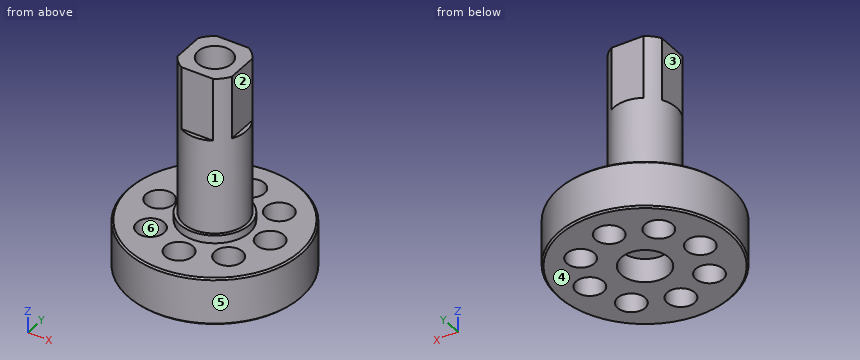
from build123d import *

# Parameters (mm, degrees)
F0_R      = 11
F1_DEPTH  = 6
F2_R      = 4
F3_DEPTH  = 21
F4_R      = 4.4
F5_DEPTH  = 1
F6_W      = 10
F6_H      = 10
F6_W_2    = 6.9
F6_H_2    = 6.9
F7_DEPTH  = 8
F8_R      = 1.75
F9_DEPTH  = 25
F11_SIZE  = 0.2
F12_R     = 2.15
F13_DEPTH = 10
F10_R     = 3
F14_DEPTH = 3


with BuildPart() as f1:
    # F0 (on Top) → F1 (new body)
    with BuildSketch(Plane.XY):
        Circle(F0_R)
    extrude(amount=F1_DEPTH)

    # F2 (on face) → F3 (join)
    with BuildSketch(Plane.XY.offset(6)):
        Circle(F2_R)
    extrude(amount=F3_DEPTH)

    # F4 (on face) → F5 (join)
    with BuildSketch(Plane.XY.offset(6)):
        Circle(F4_R)
    extrude(amount=F5_DEPTH)

    # F6 (on face) → F7 (cut)
    with BuildSketch(Plane.XY.offset(27)):
        Rectangle(F6_W, F6_H)
        Rectangle(F6_W_2, F6_H_2, mode=Mode.SUBTRACT)
    extrude(amount=-F7_DEPTH, mode=Mode.SUBTRACT)

    # F8 (on face) → F9 (cut)
    with BuildSketch(Plane(origin=(0, 0, 0), x_dir=(1, 0, 0), z_dir=(0, 0, -1))):
        with Locations((0, 7)):
            Circle(F8_R)
        with Locations((-4.949747, 4.949747)):
            Circle(F8_R)
        with Locations((-7, 0)):
            Circle(F8_R)
        with Locations((-4.949747, -4.949747)):
            Circle(F8_R)
        with Locations((0, -7)):
            Circle(F8_R)
        with Locations((4.949747, -4.949747)):
            Circle(F8_R)
        with Locations((7, 0)):
            Circle(F8_R)
        with Locations((4.949747, 4.949747)):
            Circle(F8_R)
    extrude(amount=-F9_DEPTH, mode=Mode.SUBTRACT)

    # F11
    f11_edges = [f1.edges().sort_by_distance(p)[0] for p in [
        (11, 0, 3),
        (-11, 0, 0),
        (-11, 0, 6),
    ]]
    chamfer(f11_edges, length=F11_SIZE)

    # F12 (on face) → F13 (cut)
    with BuildSketch(Plane.XY.offset(27)):
        Circle(F12_R)
    extrude(amount=-F13_DEPTH, mode=Mode.SUBTRACT)

    # F10 (on face) → F14 (cut)
    with BuildSketch(Plane(origin=(0, 0, 0), x_dir=(1, 0, 0), z_dir=(0, 0, -1))):
        Circle(F10_R)
    extrude(amount=-F14_DEPTH, mode=Mode.SUBTRACT)


solid = f1.part
For this review, take the finished solid that the model builds, in its own axes (mm). Face numbers are marked on the shaded views. A direction names the side the tool comes from. Round coordinates to 2 decimals unless told otherwise and drop trailing zeros. Write each loop counter-clockwise with the first axis right and the second up, starting at its lowest first coordinate (ties: lowest second). Pieces come first, ordered by that corner, then holes. Notation, with made-up numbers: (14, -39) -> (48, -39) arc R13 cw to (48, -20) -> close; hole circle Ø5 at (88, -39). An arc over 180 degrees is marked (long way). Put each result on its own line as item: value.
Q1. The part is to be moulded in two halves that separate along X. For the marked faces 4, 5 and 6, say which applies: released by +X, released by -X, zero draft, split by the parting line, or undercut.
Determined:
face 4: zero draft
face 5: split by the parting line
face 6: undercut
Q2. Clearance check with flat-ended pins moving along their axes: pin 1 Ø2 at (x, y) = (-0.5, 0.5) entering from +Z; pin 2 Ø3 at (x, z) = (0.5, 22.5) entering from -Y; pin 3 Ø12 at (x, z) = (5, 21.5) entering from +Y; pin 4 Ø3 at (x, y) = (-4.95, -4.95) entering from -Z. State where each tip first meets the part, or that it passes through.
Determined:
pin 1: stops at z = 17
pin 2: stops at y = -3.45
pin 3: stops at y = 4
pin 4: passes through
Q3. Machinability: for the marked faces 1, 2 and 3, which of the approach directions +Z, -Z, +X, -X, +Y, -Y give a long, thin tool a straight path to every point of the face, cutting with its end or side? Answer none if there is none.
Determined:
face 1: +Z
face 2: +Z, +X, +Y, -Y
face 3: +Z, -X, +Y, -Y
Q4. To check wall thickness, follow L1, parallel to Y at x = 0, z = 4.75; L2, parallel to Y at x = 7, z = 1.9; L3, parallel to Z at x = -2.75, y = -6.25. State the ranges of each line that lie inside material, in increasing order. Write a range as [from, to].
Determined:
L1: y = [-11, -8.75], [-5.25, 5.25], [8.75, 11]
L2: y = [-8.49, -1.75], [1.75, 8.49]
L3: z = [0, 6]
Q5. Consider section A-A on z = 24.25. State the section outline as (x, y) points.
Determined:
outline: (-3.45, -2.02) arc R4 ccw to (-2.02, -3.45) -> (2.02, -3.45) arc R4 ccw to (3.45, -2.02) -> (3.45, 2.02) arc R4 ccw to (2.02, 3.45) -> (-2.02, 3.45) arc R4 ccw to (-3.45, 2.02) -> close; hole circle Ø4.3 at (0, 0)
Q6. Consider section B-B on x = 0. Give the number of separate pieces and of enclosed holes in the cut face, and give its area (3 significant figures).
Determined:
separate pieces: 3
enclosed holes: 0
area: 189 mm^2
